Autodesk Inventor part; units mm, degrees
ref_plane "YZ Plane" through (0, 0, 0) normal (1, 0, 0) x (0, 1, 0)
ref_plane "XZ Plane" through (0, 0, 0) normal (0, 1, 0) x (-1, 0, 0)
ref_plane "XY Plane" through (0, 0, 0) normal (0, 0, 1) x (1, 0, 0)
sketch "Sketch4" plane through (0, 0, 0) normal (0, 1, 0) x (-1, 0, 0)
  line L0 (9.525, 25.4) -> (-9.525, 25.4)
  line L1 (-9.525, 25.4) -> (-9.525, -25.4)
  line L2 (-9.525, -25.4) -> (9.525, -25.4)
  line L3 (9.525, -25.4) -> (9.525, 25.4)
  line L4 (9.525, 25.4) -> (-9.525, -25.4) construction
  line L5 (-9.525, 25.4) -> (9.525, -25.4) construction
  arc A0 (-9.525, -25.4) -> (9.525, -25.4) centre (0, -16.9997) ccw
  point P0 (0, 0)
  dimension "d10" = 19.05
  dimension "d11" = 50.8
  dimension "d12" = 12.7
extrude "Extrusion2" add sketch "Sketch4" along normal blind 1.9844
sketch "Sketch5" plane through (0, 1.9844, 0) normal (0, 1, 0) x (1, 0, 0)
  point P0 (0, 0)
  point P1 (0, 15.24)
  point P2 (0, -15.24)
  dimension "d15" = 15.24
  dimension "d16" = 15.24
hole "Hole1" at (0, 1.9844, -15.24) at (0, 1.9844, 15.24) direction (0, -1, 0) diameter 6.35 depth 15.6718 tip angle 118 countersink diameter 9.525 countersink angle 82
sketch "Sketch6" plane through (-9.525, 0, 25.4) normal (0, 0, 1) x (1, 0, 0)
  line L0 (0, 1.9844) -> (19.05, 1.9844)
  line L1 (19.05, 1.9844) -> (19.05, -48.8156)
  line L2 (19.05, -48.8156) -> (0, -48.8156)
  line L3 (0, -48.8156) -> (0, 1.9844)
  arc A0 (0, -48.8156) -> (19.05, -48.8156) centre (9.525, -40.4154) ccw
  point P0 (9.525, 0)
  dimension "d24" = 19.05
  dimension "d25" = 50.8
  dimension "d28" = 12.7
extrude "Extrusion3" add sketch "Sketch6" against normal blind 1.9844
sketch "Sketch7" plane through (-9.525, 1.9844, 25.4) normal (0, 0, 1) x (1, 0, 0)
  line L0 (0, -50.8) -> (0, 0) construction
  line L1 (19.05, -1.9844) -> (19.05, -50.8) construction
  line L2 (0, 0) -> (19.05, 0) construction
  line L3 (19.05, 0) -> (19.05, -50.8) construction
  line L4 (19.05, -50.8) -> (0, -50.8) construction
  line L5 (0, -50.8) -> (0, 0) construction
  line L6 (9.525, -25.4) -> (19.05, -25.4) construction
  point P0 (9.525, -1.9844)
  point P1 (9.525, -10.16)
  point P2 (9.525, -40.64)
  dimension "d29" = 15.24
  dimension "d30" = 15.24
hole "Hole2" at (0, -8.1756, 25.4) at (0, -38.6556, 25.4) direction (0, 0, -1) diameter 6.35 depth 15.6718 tip angle 118 countersink diameter 9.525 countersink angle 82
properties part number "CornerBrace"
Design review of the part built by this model. Coordinates are the model's own, in mm. A direction names the side the tool comes from. Give positions to 0.01 mm unless a question says otherwise; leave off trailing zeros. Loops run counter-clockwise (first coordinate to the right, second up) from the corner with the lowest first, then second, coordinate; pieces in that order, holes last. Notation, with made-up numbers: M 45.25,34.25 L 76.25,34.25 A20 ccw 76.25,39.25 Z; hole C 27.25,65.5 d10. An arc over 180 degrees is marked long. Write item = value, one per line.
Q1. We need section A-A (x = 0). Count the separate pieces of the cut face and the enclosed holes in it, plus the area to 3 significant figures.
Output values:
separate_pieces = 5
enclosed_holes = 0
area = 153 mm^2
Q2. Insertion check: pin 1 (6 mm diameter, centred on x = -4, y = -16.5, fed in from -Z); pin 2 (12 mm diameter, centred on y = -13, z = 14, fed in from -X); pin 3 (10 mm diameter, centred on x = 0, z = -15.24, fed in from -Y). Each pin has a flat end and moves straight along its axis. Give the tip position at first contact, or say it passes through.
Output values:
pin_1 = 23.42
pin_2 = through
pin_3 = 0
Q3. We need section D-D (z = -5). Give the boundary of the cut face in (x, y) (3 decimals), plus the area to 3 significant figures.
Output values:
outline = M -9.525,0 L 9.525,0 L 9.525,1.984 L -9.525,1.984 Z
area = 37.8 mm^2
Q4. To check wall thickness, follow line 1 (Y direction, x = 0, z = 23.5); line 2 (Z direction, x = 0, y = 0.15) (3 decimals); line 3 (Z direction, x = 0.25, y = 0.5). State the ranges of each line that lie inside material, in increasing order. Write a range as [from, to].
Output values:
line_1 = [-53.12, -41.83], [-35.48, -11.35], [-5, 1.98]
line_2 = [-29.7, -18.415], [-12.065, 12.065], [18.415, 25.4]
line_3 = [-29.7, -18.7], [-11.78, 11.78], [18.7, 25.4]
Q5. Draft analysis for pull direction Z (two halves, no side actions). For faces 1 (the cylindrical face through (-0.151, -53.114, 24.422)), 2 (the conical face through (0.144, 0.272, 11.969)), 3 (the flat face through (0, -26, 23.416)), 4 (the conical face through (2.2, 0.3, -17.7)), state which applies: +Z half, -Z half, draft (parallel to the pull), parting line (faces both ways), or undercut.
Output values:
face_1 = draft
face_2 = undercut
face_3 = -Z half
face_4 = undercut
Q6. We need section C-C (y = -26). Give the boundary of the cut face in (x, z) (3 decimals).
Output values:
outline = M -9.525,23.416 L 9.525,23.416 L 9.525,25.4 L -9.525,25.4 Z
Q7. For faces 5 (the flat face through (0, 0, -3)), 6 (the flat face through (9.525, 1, 11)), list the 3-axis set-ups (+Z, -Z, +X, -X, +Y, -Y) from which the entire face can be reached by the end or side of a thin tool; tool diameter is ignored.
Output values:
face_5 = -Z, +X, -X, -Y
face_6 = +Z, -Z, +X, +Y, -Y
